Geometry: final body of the model. Coordinates: model frame, mm. Face numbers are marked on the shaded views. A direction names the side the tool comes from. Round coordinates to 2 decimals unless told otherwise and drop trailing zeros. Order: outer loops, then holes, each group sorted by start corner. A loop starts at its lowest first (then second) coordinate and runs counter-clockwise, first axis right, second up. Notation, with made-up numbers: (-7.75, 51.25) -> (12.25, 51.25) arc R21 ccw to (12.25, 69.25) -> close; hole circle Ø2 at (83, 85.5). An arc over 180 degrees is marked (long way). Put each result on its own line as item: value.
```python
from build123d import *

# Parameters (mm, degrees)
F0_W     = 156.6164
F0_H     = 69.85
F1_DEPTH = 50.8
F3_DEPTH = 90.424
F4_W     = 28.712457
F4_H     = 44.847306
F5_DEPTH = 10.922
F6_W     = 1.7526
F6_H     = 6.634839
F7_DEPTH = 123.1646
F8_W     = 1.7526
F8_H     = 8.506187
F9_DEPTH = 74.7776


with BuildPart() as f1:
    # F0 (on Top) → F1 (new body)
    with BuildSketch(Plane.XY):
        Rectangle(F0_W, F0_H)
    extrude(amount=F1_DEPTH)

    # F2 (on face) → F3 (cut)
    with BuildSketch(Plane.XZ.offset(34.925)):
        Polygon((-96.243918, 45.539286), (-80.431662, 5.481581), (-59.348658, 18.553045), (-30.254111, 18.553045), (18.44763, 18.553045), (24.561701, 25.299605), (41.006446, 25.299605), (54.499563, 28.462056), (78.3082, 40.901028), (84.015772, 52.707508), (-62.089447, 67.676447), align=None)
    extrude(amount=-F3_DEPTH, mode=Mode.SUBTRACT)

    # F4 (on face) → F5 (cut)
    with BuildSketch(Plane.XY.offset(18.553045)):
        with Locations((-5.434541, 1.473863)):
            Rectangle(F4_W, F4_H)
    extrude(amount=-F5_DEPTH, mode=Mode.SUBTRACT)

    # F6 (on face) → F7 (cut)
    with BuildSketch(Plane.XZ.offset(34.925)):
        with Locations((-66.516876, 0.035381)):
            Rectangle(F6_W, F6_H)
    extrude(amount=-F7_DEPTH, mode=Mode.SUBTRACT)

    # F8 (on face) → F9 (cut)
    with BuildSketch(Plane.XZ.offset(34.925)):
        with Locations((52.404836, -0.900293)):
            Rectangle(F8_W, F8_H)
    extrude(amount=-F9_DEPTH, mode=Mode.SUBTRACT)


solid = f1.part
```
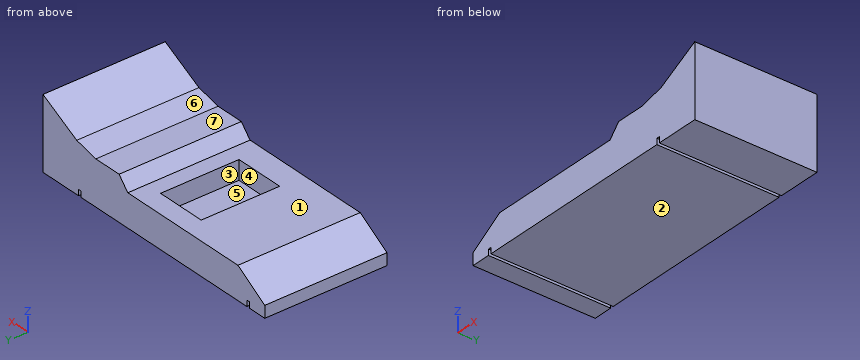
1. Draft query along X for the marked faces 4, 5, 6 and 7. Return one class per face: +X half, -X half, draft (parallel to the pull), parting line (faces both ways), or undercut.
Ans:
face 4: undercut
face 5: undercut
face 6: -X half
face 7: draft
2. Cut plane B-B on y = 11. Return loops of the section in (x, z).
Ans:
outline: (-78.31, 0) -> (-67.39, 0) -> (-67.39, 3.35) -> (-65.64, 3.35) -> (-65.64, 0) -> (51.53, 0) -> (51.53, 3.35) -> (53.28, 3.35) -> (53.28, 0) -> (78.31, 0) -> (78.31, 40.9) -> (54.5, 28.46) -> (41.01, 25.3) -> (24.56, 25.3) -> (18.45, 18.55) -> (8.92, 18.55) -> (8.92, 7.63) -> (-19.79, 7.63) -> (-19.79, 18.55) -> (-59.35, 18.55) -> (-78.31, 6.8) -> close
3. Cut plane C-C on z = 15. Return loops of the section in (x, y) (3 decimals).
Ans:
outline: (-65.079, -34.925) -> (78.308, -34.925) -> (78.308, 34.925) -> (-65.079, 34.925) -> close; hole (-19.791, -20.95) -> (8.922, -20.95) -> (8.922, 23.898) -> (-19.791, 23.898) -> close
4. Cut plane A-A on x = -2.5. Return loops of the section in (y, z) (3 decimals).
Ans:
outline: (-34.925, 0) -> (34.925, 0) -> (34.925, 18.553) -> (23.898, 18.553) -> (23.898, 7.631) -> (-20.95, 7.631) -> (-20.95, 18.553) -> (-34.925, 18.553) -> close
5. Contact query for flat-ended pins moving along their axis: P1, Ø3.5, axis at y = 4.5, z = 11.5, coming from the -X side; P2, Ø12, axis at x = -43, y = -13, coming from the +Z side; P3, Ø5, axis at x = 31, y = 6.5, coming from the +Z side. Output: stop coordinate, or through.
Ans:
P1: x = -73.55
P2: z = 18.55
P3: z = 25.3
6. Cut plane D-D on y = -24. Return loops of the section in (x, z), and give its area (3 significant figures).
Ans:
outline: (-78.31, 0) -> (-67.39, 0) -> (-67.39, 3.35) -> (-65.64, 3.35) -> (-65.64, 0) -> (51.53, 0) -> (51.53, 3.35) -> (53.28, 3.35) -> (53.28, 0) -> (78.31, 0) -> (78.31, 40.9) -> (54.5, 28.46) -> (41.01, 25.3) -> (24.56, 25.3) -> (18.45, 18.55) -> (-59.35, 18.55) -> (-78.31, 6.8) -> close
area: 3,410 mm²
7. Set-up query: the marked faces 1, 2 and 3. Return all of +Z, -Z, +X, -X, +Y, -Y with unobstructed straight access to the full face (end or side cutting, diameter ignored); none if empty.
Ans:
face 1: +Z, -X, +Y, -Y
face 2: -Z, +X, -X, +Y, -Y
face 3: +Z
8. Material intervals for probe 1 along X at (y, z) = (-8, 3); probe 2 along Z at (x, y) = (10.5, -25.5); probe 3 along Z at (x, y) = (-12, -8), sorted ascending.
Ans:
probe 1: -78.31 to -67.39, -65.64 to 51.53, 53.28 to 78.31
probe 2: 0 to 18.55
probe 3: 0 to 7.63
